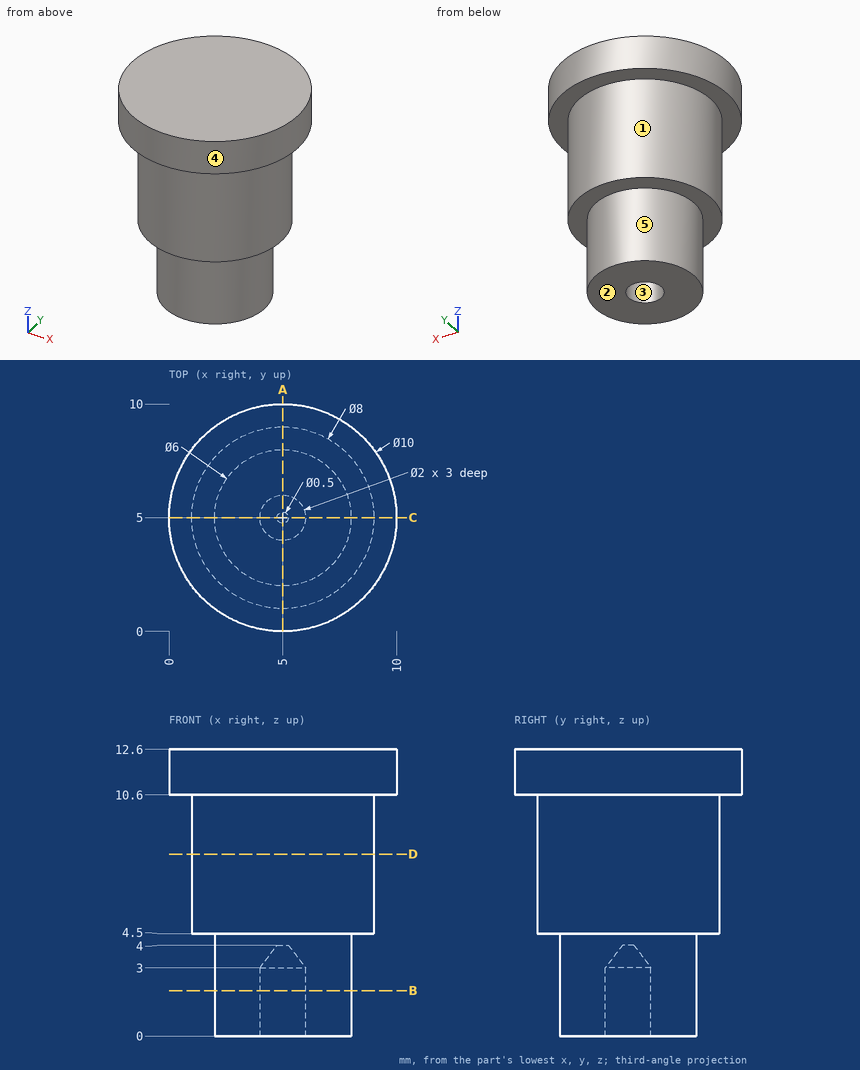
Input: dimensioned drawing with shaded views. Units: mm. Origin: part minimum x, y, z. A direction names the side the tool comes from. Give positions to 0.01 mm unless a question says otherwise; leave off trailing zeros. Write each loop counter-clockwise with the first axis right and the second up, starting at its lowest first coordinate (ties: lowest second). Pieces come first, ordered by that corner, then holes. Notation, with made-up numbers: (70.5, -14) -> (128.5, -14) arc R11 cw to (128.5, -8) -> close; hole circle Ø8 at (84.25, 88.5). An arc over 180 degrees is marked (long way). Answer as a JSON object with one key per item and string values.
1. Cut plane D-D on z = 8. Output: boundary loops of the cut face in (x, y), and give its area (3 significant figures).
Ans:
{"outline": "circle Ø8 at (5, 5)", "area": "50.3 mm^2"}
2. Ray query, probe 1 along Y at (x, z) = (5, 2.2); probe 2 along Z at (x, y) = (8.75, 7); probe 3 along Z at (x, y) = (1.5, 6.25). Return the intervals inside material, ascending. Write a range as from..to.
Ans:
{"probe 1": "y = 2..4, 6..8", "probe 2": "z = 10.6..12.6", "probe 3": "z = 4.5..12.6"}
3. Cut plane A-A on x = 5. Output: boundary loops of the cut face in (y, z), and give its area (4 significant figures).
Ans:
{"outline": "(0, 10.6) -> (1, 10.6) -> (1, 4.5) -> (2, 4.5) -> (2, 0) -> (4, 0) -> (4, 3) -> (4.75, 4) -> (5.25, 4) -> (6, 3) -> (6, 0) -> (8, 0) -> (8, 4.5) -> (9, 4.5) -> (9, 10.6) -> (10, 10.6) -> (10, 12.6) -> (0, 12.6) -> close", "area": "88.55 mm^2"}
4. Contact query for flat-ended pins moving along their axis: pin 1 (3 mm diameter, centred on x = 5, y = 5, fed in from -Z); pin 2 (6 mm diameter, centred on y = 3.5, z = 3.5, fed in from -X); pin 3 (4 mm diameter, centred on x = 6, z = 5, fed in from +Y); pin 4 (6 mm diameter, centred on y = 1.5, z = 8.5, fed in from -X). Output: stop coordinate, or through.
Ans:
{"pin 1": "stops at z = 0", "pin 2": "stops at x = 1", "pin 3": "stops at y = 9", "pin 4": "stops at x = 0.19"}
5. Mould query, pull axis X, two halves, no side actions, for the marked faces 1, 2 and 3. Classes: pulls with the +X half, pulls with the -X half, needs draft (parallel to the pull), parting line crosses it, or undercut.
Ans:
{"face 1": "parting line crosses it", "face 2": "needs draft", "face 3": "undercut"}
6. Access query for the marked faces 4 and 5. Directions: +Z, -Z, +X, -X, +Y, -Y. A direction counts if a zero-diameter tool reaches every point of the face in a straight line with its end or side. Return the directions, or none.
Ans:
{"face 4": "+Z, -Z", "face 5": "-Z"}
7. Cut plane B-B on z = 2. Output: boundary loops of the cut face in (x, y), and give its area (3 significant figures).
Ans:
{"outline": "circle Ø6 at (5, 5); hole circle Ø2 at (5, 5)", "area": "25.1 mm^2"}
